Autodesk Inventor part; units mm, degrees
ref_plane "YZ Plane" through (0, 0, 0) normal (1, 0, 0) x (0, 1, 0)
ref_plane "XZ Plane" through (0, 0, 0) normal (0, 1, 0) x (-1, 0, 0)
ref_plane "XY Plane" through (0, 0, 0) normal (0, 0, 1) x (1, 0, 0)
sketch "Sketch1" plane through (0, 0, 0) normal (0, 1, 0) x (-1, 0, 0)
  line L0 (0, 0) -> (26.2, 0)
  line L1 (26.2, 0) -> (26.2, -33.5)
  line L2 (26.2, -33.5) -> (0, -33.5)
  line L3 (0, -33.5) -> (0, 0)
  dimension "d0" = 26.2
  dimension "d1" = 33.5
extrude "Extrusion1" add sketch "Sketch1" along normal blind 3
sketch "Sketch2" plane through (0, 3, 0) normal (0, 1, 0) x (1, 0, 0)
  line L0 (0, 33.5) -> (-26.2, 33.5)
  line L1 (-26.2, 33.5) -> (0, 33.5)
  line L2 (0, 33.5) -> (0, 30.5)
  line L3 (0, 30.5) -> (-26.2, 30.5)
  line L4 (-26.2, 30.5) -> (-26.2, 33.5)
  point P0 (0, 0)
  dimension "d4" = 26.2
  dimension "d5" = 3
extrude "Extrusion2" add sketch "Sketch2" along normal blind 30.5
fillet "Fillet1" radius 3 1 edges at (-13.1, 0, -33.5)
fillet "Fillet2" radius 13.1 2 edges at (0, 33.5, -32) (-26.2, 33.5, -32)
fillet "Fillet3" radius 1 2 edges at (-26.2, 1.5, 0) (0, 1.5, 0)
sketch "Sketch3" plane through (0, 3, 0) normal (0, 1, 0) x (1, 0, 0)
  circle A0 centre (-13.1, 15) radius 5
  line L0 (0, 1) -> (0, 30.5)
  line L1 (-25.2, 0) -> (-1, 0)
  circle A1 centre (-21.1, 8) radius 1.75
  line L2 (-26.2, 30.5) -> (-26.2, 1)
  circle A2 centre (-5.1, 8) radius 1.75
  circle A3 centre (-21.1, 22) radius 1.75
  circle A4 centre (-5.1, 22) radius 1.75
  point P0 (0, 0)
  dimension "d11" = 10
  dimension "d12" = 13.1
  dimension "d13" = 15
  dimension "d14" = 3.5
  dimension "d15" = 7
  dimension "d16" = 5.1
  dimension "d19" = 16
  dimension "d22" = 14
extrude "Extrusion3" cut sketch "Sketch3" against normal through all
sketch "Sketch4" plane through (0, 3, -33.5) normal (0, 0, -1) x (-1, 0, 0)
  circle A0 centre (13.1, 17.5) radius 4
  arc A1 (26.2, 17.4) -> (0, 17.4) centre (13.1, 17.4) ccw
  line L0 (0, 0) -> (0, 17.4)
  circle A2 centre (4.6, 17.5) radius 1.75
  circle A3 centre (21.6, 17.5) radius 1.75
  point P0 (0, -3)
  point P1 (13.1, 30.5)
  dimension "d27" = 8
  dimension "d28" = 13
  dimension "d32" = 13.1
  dimension "d33" = 3.5
  dimension "d34" = 4.6
  dimension "d35" = 3.5
  dimension "d36" = 17
extrude "Extrusion4" cut sketch "Sketch4" against normal through all
properties part number "suporte"
Verification items for the finished model (mm, model axes). A direction names the side the tool comes from. Give positions to 0.01 mm unless a question says otherwise; leave off trailing zeros. Order: outer loops, then holes, each group sorted by start corner. A loop starts at its lowest first (then second) coordinate and runs counter-clockwise, first axis right, second up. Notation, with made-up numbers: (52.5, 75.5) -> (83.5, 75.5) arc R25 cw to (83.5, 91.5) -> close; hole circle Ø1 at (-39, 26). An arc over 180 degrees is marked (long way). One line per item, written item: value.
(1) Tool access check on faces 4 (the face through (0, 2.6, -23.3)), 5 (the face through (-7, 3, -15)). Record the directions out of +Z, -Z, +X, -X, +Y, -Y that give a thin tool (end or side, any length) a straight path to the whole face; none if there is none.
Final values:
face 4: +Z, -Z, +X, +Y, -Y
face 5: +Z, +X, -X, +Y
(2) Gauge pin test, flat ends, axial feed: pin 1 (8 mm diameter, centred on x = -15, y = 11, fed in from +Z); pin 2 (3 mm diameter, centred on x = -21.1, z = -8, fed in from +Y); pin 3 (3 mm diameter, centred on x = -21.5, z = -4, fed in from +Y). Record the tip position at first contact, or that the pin passes through.
Final values:
pin 1: z = -30.5
pin 2: through
pin 3: y = 3
(3) Sectioned sample at A-A on z = -15. Record the cut outline in (x, y).
Final values:
outline: (-26.2, 0) -> (-18.1, 0) -> (-18.1, 3) -> (-26.2, 3) -> close; (-8.1, 0) -> (0, 0) -> (0, 3) -> (-8.1, 3) -> close
(4) Sectioned sample at D-D on z = -22. Record the cut outline in (x, y).
Final values:
outline: (-26.2, 0) -> (-22.85, 0) -> (-22.85, 3) -> (-26.2, 3) -> close; (-19.35, 0) -> (-6.85, 0) -> (-6.85, 3) -> (-19.35, 3) -> close; (-3.35, 0) -> (0, 0) -> (0, 3) -> (-3.35, 3) -> close
(5) Sectioned sample at B-B on x = -12.5. Record the cut outline in (y, z).
Final values:
outline: (0, -30.5) arc R3 ccw to (3, -33.5) -> (16.55, -33.5) -> (16.55, -30.5) -> (3, -30.5) -> (3, -19.96) -> (0, -19.96) -> close; (0, -10.04) -> (3, -10.04) -> (3, 0) -> (0, 0) -> close; (24.45, -33.5) -> (33.49, -33.5) -> (33.49, -30.5) -> (24.45, -30.5) -> close
(6) Sectioned sample at C-C on x = -5.1. Record the cut outline in (y, z), then the cut area to 3 significant figures.
Final values:
outline: (0, -30.5) arc R3 ccw to (3, -33.5) -> (18.82, -33.5) -> (18.82, -30.5) -> (3, -30.5) -> (3, -23.75) -> (0, -23.75) -> close; (0, -20.25) -> (3, -20.25) -> (3, -9.75) -> (0, -9.75) -> close; (0, -6.25) -> (3, -6.25) -> (3, 0) -> (0, 0) -> close; (22.18, -33.5) -> (30.77, -33.5) -> (30.77, -30.5) -> (22.18, -30.5) -> close
area: 151 mm^2
(7) Scan lines: line 1 along X through (y, z) = (0.8, -8); line 2 along Z through (x, y) = (-5.1, 1.5); line 3 along Y through (x, z) = (-1.5, -18). Record each from-to range of solid material in increasing order. Write a range as [from, to].
Final values:
line 1: [-26.2, -22.85], [-19.35, -6.85], [-3.35, 0]
line 2: [-33.1, -23.75], [-20.25, -9.75], [-6.25, 0]
line 3: [0, 3]
(8) Draft check along X on faces 1 (the face through (-10.15, 23.2, -32.02)), 2 (the face through (-7, 0, -15)), 3 (the face through (-0.301, 1.521, -0.285)). Enter one of: pulls with the +X half, pulls with the -X half, needs draft (parallel to the pull), parting line crosses it, or undercut.
Final values:
face 1: undercut
face 2: needs draft
face 3: pulls with the +X half
